Here's how the part is built. I have some questions about the finished solid (model axes, mm). Face numbers are marked on the shaded views. A direction names the side the tool comes from. Coordinates: 2 decimals unless noted, no trailing zeros. Write each loop counter-clockwise with the first axis right and the second up, starting at its lowest first coordinate (ties: lowest second). Pieces come first, ordered by that corner, then holes.
Item 1: If we section it at B-B (z = 5.25): Please give me the cut outline in (x, y).
Item 2: I'm going to push flat-ended pins straight in: pin 1 Ø3 at (x, z) = (41.5, 1.5) entering from -Y; pin 2 Ø1 at (x, z) = (30.5, 2) entering from +Y. Where does each tip first touch, or does it pass through?
Item 3: If I drill on line 1 (X direction, y = 33, z = 2.75); line 2 (Y direction, x = 53, z = 2.25); line 3 (X direction, y = 36, z = 6), over which ranges is the centre line in solid material (lowest first)?
Item 4: We'd pull the mould along X, two halves only. Please class the marked faces 4 and 5: +X half, -X half, draft (parallel to the pull), parting line (faces both ways), or undercut.
Item 5: If we section it at C-C (x = 37): Please give me the cut outline in (y, z).
Item 6: For the marked faces 1, 2 and 3, which set-ups out of +Z, -Z, +X, -X, +Y, -Y let a thin tool reach every point of the face, with its end or its side?
Item 7: If we section it at A-A (y = 31.5): Please give me the cut outline in (x, z), then the cut area to 3 significant figures.
from build123d import *

# Parameters (mm, degrees)
BOSS_EXTRUDE2_DEPTH = 6.35


with BuildPart() as part:
    # Sketch3 → Boss-Extrude2 (new body)
    with BuildSketch(Plane.XY):
        with BuildLine():
            Line((0, 0), (0, 38.1))
            Line((0, 38.1), (1.27, 38.1))
            ThreePointArc((1.27, 38.1), (4.862102448, 36.612102448), (6.35, 33.02))
            Line((6.35, 33.02), (6.35, 27.94))
            ThreePointArc((6.35, 27.94), (7.837897552, 24.347897552), (11.43, 22.86))
            Line((11.43, 22.86), (82.55, 22.86))
            ThreePointArc((82.55, 22.86), (86.142102448, 24.347897552), (87.63, 27.94))
            Line((87.63, 27.94), (87.63, 33.02))
            ThreePointArc((87.63, 33.02), (89.117897552, 36.612102448), (92.71, 38.1))
            Line((92.71, 38.1), (93.98, 38.1))
            Line((93.98, 38.1), (93.98, 0))
            Line((93.98, 0), (92.71, 0))
            ThreePointArc((92.71, 0), (89.117897552, 1.487897552), (87.63, 5.08))
            Line((87.63, 5.08), (87.63, 10.033))
            ThreePointArc((87.63, 10.033), (86.142102448, 13.625102448), (82.55, 15.113))
            Line((82.55, 15.113), (11.43, 15.113))
            ThreePointArc((11.43, 15.113), (7.837897552, 13.625102448), (6.35, 10.033))
            Line((6.35, 10.033), (6.35, 5.08))
            ThreePointArc((6.35, 5.08), (4.862102448, 1.487897552), (1.27, 0))
            Line((1.27, 0), (0, 0))
        make_face()
    extrude(amount=BOSS_EXTRUDE2_DEPTH)


solid = part.part
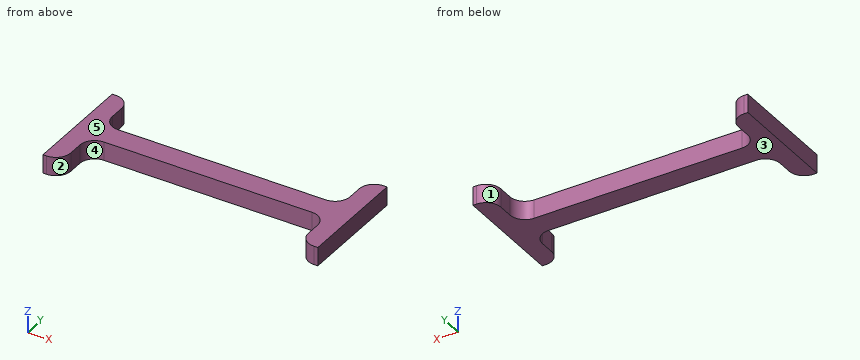
Answer list:
1. outline: (0, 0) - (1.27, 0) arc R5.08 ccw to (6.35, 5.08) - (6.35, 10.03) arc R5.08 cw to (11.43, 15.11) - (82.55, 15.11) arc R5.08 cw to (87.63, 10.03) - (87.63, 5.08) arc R5.08 ccw to (92.71, 0) - (93.98, 0) - (93.98, 38.1) - (92.71, 38.1) arc R5.08 ccw to (87.63, 33.02) - (87.63, 27.94) arc R5.08 cw to (82.55, 22.86) - (11.43, 22.86) arc R5.08 cw to (6.35, 27.94) - (6.35, 33.02) arc R5.08 ccw to (1.27, 38.1) - (0, 38.1) - close
2. pin 1: stops at y = 15.11
2. pin 2: stops at y = 22.86
3. line 1: x = 0 to 6.35, 87.63 to 93.98
3. line 2: y = 15.11 to 22.86
3. line 3: x = 0 to 5.38, 88.6 to 93.98
4. face 4: undercut
4. face 5: draft
5. outline: (15.11, 0) - (22.86, 0) - (22.86, 6.35) - (15.11, 6.35) - close
6. face 1: +Z, -Z, +Y
6. face 2: +Z, -Z, -Y
6. face 3: -Z, +X, -X, +Y, -Y
7. outline: (0, 0) - (6.35, 0) - (6.35, 6.35) - (0, 6.35) - close; (87.63, 0) - (93.98, 0) - (93.98, 6.35) - (87.63, 6.35) - close
7. area: 80.6 mm2
